Check sheet for the modelled part. Datum: model origin and axes. Units: mm. A direction names the side the tool comes from. Coordinates: 2 decimals unless noted, no trailing zeros. Loops run counter-clockwise (first coordinate to the right, second up) from the corner with the lowest first, then second, coordinate; pieces in that order, holes last. Notation, with made-up numbers: (-8, -16) - (17, -16) arc R25 cw to (17, 22) - close; hole circle Ø5 at (47, 3.5). An arc over 180 degrees is marked (long way). Write each question's results on one line, items separated by ' | '. Start each with the question number.
1. Cross-section at A-A (z = 24.9). Record the cut outline in (x, y).
2. Gauge pin test, flat ends, axial feed: P1, Ø1.5, axis at y = 40.5, z = 17.5, coming from the -X side; P2, Ø4, axis at x = 12.5, z = 32.5, coming from the -Y side; P3, Ø1.6, axis at x = 25.5, z = 37.5, coming from the -Y side; P4, Ø6, axis at x = 10.5, z = 8, coming from the +Y side. Record the tip position at first contact, or that the pin passes through.
3. Cross-section at B-B (x = 25). Record the cut outline in (y, z).
4. Cross-section at D-D (z = 33). Record the cut outline in (x, y).
5. Thickness scan on line 1 (Z direction, x = 16, y = 154.5); line 2 (Y direction, x = 24, z = 29.5). Record the ranges inside material, lowest first. Write a range as [from, to].
6. Cross-section at C-C (y = 109.5). Record the cut outline in (x, z), and give its area (3 significant figures).
7. Tool access check on faces 1 (the face through (25, 174, 6)), 2 (the face through (25, 93, 36.25)), 3 (the face through (25, 94, 0)). Record the directions out of +Z, -Z, +X, -X, +Y, -Y that give a thin tool (end or side, any length) a straight path to the whole face; none if there is none.
8. Draft check along X on faces 4 (the face through (46.83, 5.07, 2.34)), 5 (the face through (25, 196, 25)), 6 (the face through (0, 94, 18)). Enter one of: released by +X, released by -X, zero draft, split by the parting line, or undercut.
```python
from build123d import *

# Parameters (mm, degrees)
F1_DEPTH  = 4.75
F2_W      = 50
F2_H      = 164
F3_DEPTH  = 31.5
F5_D      = 3.6576
F6_R      = 16.65
F7_DEPTH  = 14
F8_R      = 10
F9_DEPTH  = 3
F10_R     = 3.75
F11_DEPTH = 5


with BuildPart() as f1:
    # F0 (on Top) → F1 (new body)
    with BuildSketch(Plane.XY):
        with BuildLine():
            ThreePointArc((0, 2), (0.5857864376, 0.5857864376), (2, 0))
            Line((2, 0), (48, 0))
            ThreePointArc((48, 0), (49.4142135624, 0.5857864376), (50, 2))
            Line((50, 2), (50, 183))
            ThreePointArc((50, 183), (49.4142135624, 184.4142135624), (48, 185))
            Line((48, 185), (2, 185))
            ThreePointArc((2, 185), (0.5857864376, 184.4142135624), (0, 183))
            Line((0, 183), (0, 2))
        make_face()
    extrude(amount=F1_DEPTH)

    # F2 (on face) → F3 (join)
    with BuildSketch(Plane.XY.offset(4.75)):
        with Locations((25, 92)):
            Rectangle(F2_W, F2_H)
    extrude(amount=F3_DEPTH)

    # F5 (through all)
    with Locations(Plane.XY.offset(4.75)):
        with Locations((4.9975, 179.0077), (45.0025, 179.0077), (4.9975, 4.9923), (45.0025, 4.9923)):
            Hole(F5_D / 2)

    # F6 (on face) → F7 (join)
    with BuildSketch(Plane(origin=(0, 174, 0), x_dir=(-1, 0, 0), z_dir=(0, 1, 0))):
        with Locations((-25, 24.9)):
            Circle(F6_R)
    extrude(amount=F7_DEPTH)

    # F8 (on face) → F9 (join)
    with BuildSketch(Plane(origin=(0, 188, 0), x_dir=(-1, 0, 0), z_dir=(0, 1, 0))):
        with Locations((-25, 24.9)):
            Circle(F8_R)
    extrude(amount=F9_DEPTH)

    # F10 (on face) → F11 (join)
    with BuildSketch(Plane(origin=(0, 191, 0), x_dir=(-1, 0, 0), z_dir=(0, 1, 0))):
        with Locations((-25, 24.9)):
            Circle(F10_R)
    extrude(amount=F11_DEPTH)


solid = f1.part
```
Established:
1) outline: (0, 10) - (50, 10) - (50, 174) - (41.65, 174) - (41.65, 188) - (35, 188) - (35, 191) - (28.75, 191) - (28.75, 196) - (21.25, 196) - (21.25, 191) - (15, 191) - (15, 188) - (8.35, 188) - (8.35, 174) - (0, 174) - close
2) P1: x = 0 | P2: y = 10 | P3: y = 174 | P4: y = 174
3) outline: (0, 0) - (185, 0) - (185, 4.75) - (174, 4.75) - (174, 8.25) - (188, 8.25) - (188, 14.9) - (191, 14.9) - (191, 21.15) - (196, 21.15) - (196, 28.65) - (191, 28.65) - (191, 34.9) - (188, 34.9) - (188, 41.55) - (174, 41.55) - (174, 36.25) - (10, 36.25) - (10, 4.75) - (0, 4.75) - close
4) outline: (0, 10) - (50, 10) - (50, 174) - (39.55, 174) - (39.55, 188) - (30.86, 188) - (30.86, 191) - (19.14, 191) - (19.14, 188) - (10.45, 188) - (10.45, 174) - (0, 174) - close
5) line 1: [0, 36.25] | line 2: [10, 191]
6) outline: (0, 0) - (50, 0) - (50, 36.25) - (0, 36.25) - close | area: 1,810 mm^2
7) face 1: +Y | face 2: +Z, +X, -X, -Y | face 3: -Z, +X, -X, +Y, -Y
8) face 4: undercut | face 5: zero draft | face 6: released by -X
